Verification items for the finished model (mm, model axes). Coordinates: 2 decimals unless noted, no trailing zeros. Loops run counter-clockwise (first coordinate to the right, second up) from the corner with the lowest first, then second, coordinate; pieces in that order, holes last. Notation, with made-up numbers: (11.5, -28) - (28.5, -28) arc R35 ccw to (28.5, 4) - close; hole circle Ø11 at (17, 21.5). An arc over 180 degrees is marked (long way). Answer as CSV lines item,"result". Start each with the question number.
1. Material ranges on line 1 (Y direction, x = 55, z = -1.8); line 2 (Y direction, x = 38.5, z = -3.55), recorded low to high. Write a range as [from, to].
2. Cross-section at C-C (y = 1.5). State how many separate pieces and enclosed holes the cut face has, plus the area to 3 significant figures.
3. Cross-section at A-A (x = -44). Enter the section's corners in (y, z), plus the area to 3 significant figures.
4. Cross-section at B-B (y = 13). Enter the section's corners in (x, z).
```python
from build123d import *

# Parameters (mm, degrees)
ESQUISSE1_W        = 140
ESQUISSE1_H        = 50
ESQUISSE1_R        = 1.55
ESQUISSE1_W_2      = 10
ESQUISSE1_H_2      = 12
BOSS_EXTRU_1_DEPTH = 5


with BuildPart() as part:
    # Esquisse1 → Boss.-Extru.1 (new body)
    with BuildSketch(Plane.XY):
        Rectangle(ESQUISSE1_W, ESQUISSE1_H)
        with Locations((-55, -13)):
            Circle(ESQUISSE1_R, mode=Mode.SUBTRACT)
        with Locations(Location((-55, 13, 0), (0, 0, 180))):
            Circle(ESQUISSE1_R, mode=Mode.SUBTRACT)
        with Locations(Location((55, -13, 0), (0, 0, 180))):
            Circle(ESQUISSE1_R, mode=Mode.SUBTRACT)
        with Locations((55, 13)):
            Circle(ESQUISSE1_R, mode=Mode.SUBTRACT)
        with Locations((13.97, -2)):
            Rectangle(ESQUISSE1_W_2, ESQUISSE1_H_2, mode=Mode.SUBTRACT)
        with Locations((0, -2)):
            Rectangle(ESQUISSE1_W_2, ESQUISSE1_H_2, mode=Mode.SUBTRACT)
        with Locations((27.94, -2)):
            Rectangle(ESQUISSE1_W_2, ESQUISSE1_H_2, mode=Mode.SUBTRACT)
        with Locations((41.91, -2)):
            Rectangle(ESQUISSE1_W_2, ESQUISSE1_H_2, mode=Mode.SUBTRACT)
        with Locations((55.88, -2)):
            Rectangle(ESQUISSE1_W_2, ESQUISSE1_H_2, mode=Mode.SUBTRACT)
        with Locations((-13.97, -2)):
            Rectangle(ESQUISSE1_W_2, ESQUISSE1_H_2, mode=Mode.SUBTRACT)
        with Locations((-27.94, -2)):
            Rectangle(ESQUISSE1_W_2, ESQUISSE1_H_2, mode=Mode.SUBTRACT)
        with Locations((-41.91, -2)):
            Rectangle(ESQUISSE1_W_2, ESQUISSE1_H_2, mode=Mode.SUBTRACT)
        with Locations((-55.88, -2)):
            Rectangle(ESQUISSE1_W_2, ESQUISSE1_H_2, mode=Mode.SUBTRACT)
    extrude(amount=-BOSS_EXTRU_1_DEPTH)


solid = part.part
```
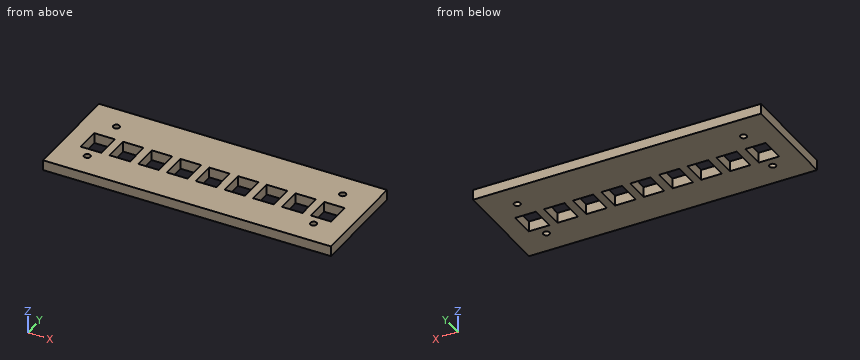
Values follow:
1,line 1,"y = [-25, -14.55], [-11.45, -8], [4, 11.45], [14.55, 25]"
1,line 2,"y = [-25, -8], [4, 25]"
2,separate pieces,"10"
2,enclosed holes,"0"
2,area,"250 mm²"
3,outline,"(-25, -5) - (-8, -5) - (-8, 0) - (-25, 0) - close; (4, -5) - (25, -5) - (25, 0) - (4, 0) - close"
3,area,"190 mm²"
4,outline,"(-70, -5) - (-56.55, -5) - (-56.55, 0) - (-70, 0) - close; (-53.45, -5) - (53.45, -5) - (53.45, 0) - (-53.45, 0) - close; (56.55, -5) - (70, -5) - (70, 0) - (56.55, 0) - close"
